Autodesk Inventor part; units mm, degrees
ref_plane "YZ Plane" through (0, 0, 0) normal (1, 0, 0) x (0, 1, 0)
ref_plane "XZ Plane" through (0, 0, 0) normal (0, 1, 0) x (-1, 0, 0)
ref_plane "XY Plane" through (0, 0, 0) normal (0, 0, 1) x (1, 0, 0)
sketch "Sketch1" plane through (0, 0, 0) normal (0, 1, 0) x (-1, 0, 0)
  line L0 (0, 0) -> (10, 0)
  line L1 (10, 0) -> (10, -128)
  line L2 (10, -128) -> (0, -128)
  line L3 (0, -128) -> (0, 0)
  line L4 (10, -128) -> (10, -163)
  line L5 (10, -163) -> (30, -163)
  line L6 (10, 0) -> (10, 35)
  line L7 (10, 35) -> (30, 35)
  line L8 (30, 35) -> (30, -163)
  dimension "d16" = 35
  dimension "d17" = 20
  dimension "d18" = 35
  dimension "d19" = 20
  dimension "d28" = 128
  dimension "d35" = 10
extrude "Extrusion1" add sketch "Sketch1" along normal blind 30
sketch "Sketch2" plane through (0, 0, 0) normal (0, -1, 0) x (1, 0, 0)
  line L0 (-30, -163) -> (-30, 35)
  line L1 (-30, -104) -> (-10, -104)
  line L2 (-10, -104) -> (-10, -24)
  line L3 (-10, -24) -> (-30, -24)
  line L4 (-30, -24) -> (-30, -104)
  line L5 (-10, 0) -> (0, 0)
  dimension "d22" = 20
  dimension "d23" = 80
  dimension "d25" = 24
extrude "Extrusion6" cut sketch "Sketch2" against normal blind 10
sketch "Sketch6" plane through (0, 0, 0) normal (0, -1, 0) x (1, 0, 0)
  line L0 (-30, -24) -> (-10, -24)
  line L1 (-10, 0) -> (0, 0)
  line L2 (-30, -24) -> (0, -24)
  line L3 (0, -24) -> (0, 0)
  line L4 (0, 0) -> (-30, 0)
  line L5 (-30, 0) -> (-30, -24)
  line L6 (-10, -104) -> (-30, -104)
  line L7 (0, 0) -> (0, -128)
  line L8 (-30, -104) -> (0, -104)
  line L9 (0, -104) -> (0, -128)
  line L10 (0, -128) -> (-30, -128)
  line L11 (-30, -128) -> (-30, -104)
extrude "Extrusion7" add sketch "Sketch6" along normal blind 30
properties part number "Tunnel_Holder"
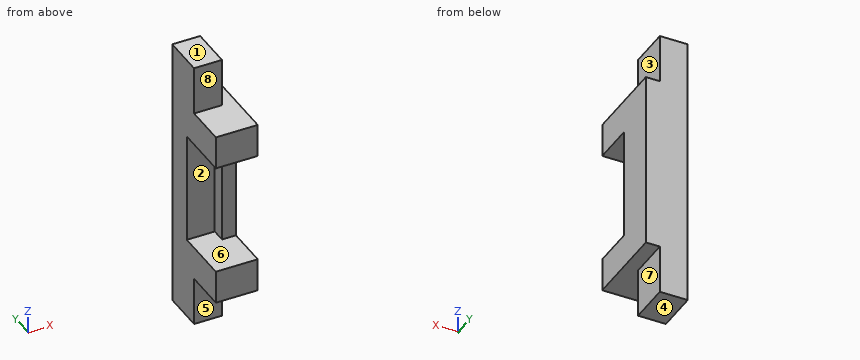
Source: CAD feature listing. Evaluate the final solid. Frame: model axes, mm. Face numbers are marked on the shaded views. A direction names the side the tool comes from. Give positions to 0.01 mm unless a question says otherwise; leave off trailing zeros. Order: outer loops, then holes, each group sorted by start corner. A loop starts at its lowest first (then second) coordinate and runs counter-clockwise, first axis right, second up. Notation, with made-up numbers: (64.5, 1.25) -> (100.5, 1.25) arc R11 ccw to (100.5, 15.25) -> close; hole circle Ø4 at (-28, 57). An arc over 180 degrees is marked (long way). Use a Markdown table: item, result.
1) Contact query for flat-ended pins moving along their axis: P1, Ø15, axis at x = -17, y = -15.5, coming from the -Z side; P2, Ø15, axis at y = 10, z = 18, coming from the +X side; P3, Ø6, axis at x = -19.5, z = -64, coming from the -Y side. Output: stop coordinate, or through.
Answer list:
| item | result |
|---|---|
| P1 | z = -128 |
| P2 | x = -10 |
| P3 | y = 10 |
2) Section query B-B, the plane x = -7.25. Return the cut outline in (y, z), then the cut area to 3 significant figures.
Answer list:
| item | result |
|---|---|
| outline | (-30, -128) -> (30, -128) -> (30, 0) -> (-30, 0) -> (-30, -24) -> (0, -24) -> (0, -104) -> (-30, -104) -> close |
| area | 5,280 mm² |
3) Mould query, pull axis Z, two halves, no side actions, for the marked faces 1, 2 and 3. Classes: +Z half, -Z half, draft (parallel to the pull), parting line (faces both ways), or undercut.
Answer list:
| item | result |
|---|---|
| face 1 | +Z half |
| face 2 | undercut |
| face 3 | draft |
4) Section query C-C, the plane y = 8. Return the cut outline in (x, z), then the cut area to 3 significant figures.
Answer list:
| item | result |
|---|---|
| outline | (-30, -163) -> (-10, -163) -> (-10, -128) -> (0, -128) -> (0, 0) -> (-10, 0) -> (-10, 35) -> (-30, 35) -> (-30, -24) -> (-10, -24) -> (-10, -104) -> (-30, -104) -> close |
| area | 3,640 mm² |
5) Reachability of the marked faces 4, 5, 6, 7 and 8 from +Z, -Z, +X, -X, +Y, -Y: full face, straight path, thin tool, end or side. Return the list, or none.
Answer list:
| item | result |
|---|---|
| face 4 | -Z, +X, -X, +Y, -Y |
| face 5 | -Z, +X, -X, -Y |
| face 6 | -X, -Y |
| face 7 | -Z, +X, +Y, -Y |
| face 8 | +Z, +X, -X, -Y |
6) Section query A-A, the plane y = -23. Return the cut outline in (x, z), then the cut area to 3 significant figures.
Answer list:
| item | result |
|---|---|
| outline | (-30, -128) -> (0, -128) -> (0, -104) -> (-30, -104) -> close; (-30, -24) -> (0, -24) -> (0, 0) -> (-30, 0) -> close |
| area | 1,440 mm² |
7) Section query D-D, the plane z = -62. Return the cut outline in (x, y).
Answer list:
| item | result |
|---|---|
| outline | (-30, 10) -> (-10, 10) -> (-10, 0) -> (0, 0) -> (0, 30) -> (-30, 30) -> close |
8) Ray query, line 1 along Z through (x, y) = (-13, -14); line 2 along Z through (x, y) = (-28, 3); line 3 along X through (y, z) = (5, -30). Return the intervals inside material, ascending. Write a range as [from, to].
Answer list:
| item | result |
|---|---|
| line 1 | [-128, -104], [-24, 0] |
| line 2 | [-163, -104], [-24, 35] |
| line 3 | [-10, 0] |
